from build123d import *

# Parameters (mm, degrees)
SKETCH1_W           = 465.838
SKETCH1_H           = 365.232
BOSS_EXTRUDE1_DEPTH = 3.175
SKETCH2_W           = 465.838
SKETCH2_H           = 365.232
SKETCH2_W_2         = 459.488
SKETCH2_H_2         = 47.625
SKETCH2_W_3         = 89.789
SKETCH2_H_3         = 308.082
SKETCH2_W_4         = 87.632
BOSS_EXTRUDE2_DEPTH = 200.6
SKETCH4_W           = 459.488
SKETCH4_H           = 200.6
CUT_EXTRUDE1_DEPTH  = 3.175
SKETCH5_W           = 89.789
SKETCH5_H           = 308.082
SKETCH5_W_2         = 87.632
BOSS_EXTRUDE5_DEPTH = 38.1
CUT_EXTRUDE2_DEPTH  = 35
BOSS_EXTRUDE6_DEPTH = 50.8
CUT_EXTRUDE3_DEPTH  = 589.161843479
SKETCH10_W          = 34.036
SKETCH10_H          = 101.6
SKETCH10_W_2        = 50.8
SKETCH10_H_2        = 34.036
BOSS_EXTRUDE7_DEPTH = 3.175


with BuildPart() as part:
    # Sketch1 → Boss-Extrude1 (new body)
    with BuildSketch(Plane.XY):
        with Locations((-46.4825, -25.4)):
            Rectangle(SKETCH1_W, SKETCH1_H)
    extrude(amount=BOSS_EXTRUDE1_DEPTH)

    # Sketch2 → Boss-Extrude2 (add)
    with BuildSketch(Plane.XY.offset(3.175)):
        with Locations((-46.4825, -25.4)):
            Rectangle(SKETCH2_W, SKETCH2_H)
        with Locations((-46.4825, -181.0285)):
            Rectangle(SKETCH2_W_2, SKETCH2_H_2, mode=Mode.SUBTRACT)
        with Locations((138.367, 0)):
            Rectangle(SKETCH2_W_3, SKETCH2_H_3, mode=Mode.SUBTRACT)
        with Locations((45.403, 0)):
            Rectangle(SKETCH2_W_3, SKETCH2_H_3, mode=Mode.SUBTRACT)
        with Locations((-47.561, 0)):
            Rectangle(SKETCH2_W_3, SKETCH2_H_3, mode=Mode.SUBTRACT)
        with Locations((-140.525, 0)):
            Rectangle(SKETCH2_W_3, SKETCH2_H_3, mode=Mode.SUBTRACT)
        with Locations((-232.4105, 0)):
            Rectangle(SKETCH2_W_4, SKETCH2_H_3, mode=Mode.SUBTRACT)
    extrude(amount=BOSS_EXTRUDE2_DEPTH)

    # Sketch4 → Cut-Extrude1 (cut)
    with BuildSketch(Plane.XZ.offset(208.016)):
        with Locations((-46.4825, 103.475)):
            Rectangle(SKETCH4_W, SKETCH4_H)
    extrude(amount=-CUT_EXTRUDE1_DEPTH, mode=Mode.SUBTRACT)

    # Sketch5 → Boss-Extrude5 (add)
    with BuildSketch(Plane.XY.offset(203.775)):
        Polygon((186.4365, 157.216), (-279.4015, 157.216), (-279.4015, -208.016), (-276.2265, -208.016), (-276.2265, -157.216), (183.2615, -157.216), (183.2615, -208.016), (186.4365, -208.016), align=None)
        with Locations((-140.525, 0)):
            Rectangle(SKETCH5_W, SKETCH5_H, mode=Mode.SUBTRACT)
        with Locations((-47.561, 0)):
            Rectangle(SKETCH5_W, SKETCH5_H, mode=Mode.SUBTRACT)
        with Locations((45.403, 0)):
            Rectangle(SKETCH5_W, SKETCH5_H, mode=Mode.SUBTRACT)
        with Locations((138.367, 0)):
            Rectangle(SKETCH5_W, SKETCH5_H, mode=Mode.SUBTRACT)
        with Locations((-232.4105, 0)):
            Rectangle(SKETCH5_W_2, SKETCH5_H, mode=Mode.SUBTRACT)
    extrude(amount=BOSS_EXTRUDE5_DEPTH)

    # Sketch7 → Cut-Extrude2 (cut)
    with BuildSketch(Plane.XY.offset(241.875)):
        Polygon((-185.4195, -154.041), (-185.4195, 154.041), (-188.5945, 154.041), (-188.5945, -154.041), (-276.2265, -154.041), (-276.2265, -157.216), (183.2615, -157.216), (183.2615, -154.041), (93.4725, -154.041), (93.4725, 154.041), (90.2975, 154.041), (90.2975, -154.041), (0.5085, -154.041), (0.5085, 154.041), (-2.6665, 154.041), (-2.6665, -154.041), (-92.4555, -154.041), (-92.4555, 154.041), (-95.6305, 154.041), (-95.6305, -154.041), align=None)
    extrude(amount=-CUT_EXTRUDE2_DEPTH, mode=Mode.SUBTRACT)

    # Sketch8 → Boss-Extrude6 (add)
    with BuildSketch(Plane.XY.offset(241.875)):
        Polygon((183.2615, 154.041), (183.2615, -208.016), (186.4365, -208.016), (186.4365, 157.216), (-279.4015, 157.216), (-279.4015, -208.016), (-276.2265, -208.016), (-276.2265, 154.041), align=None)
    extrude(amount=BOSS_EXTRUDE6_DEPTH)

    # Sketch9 → Cut-Extrude3 (cut, through all)
    with BuildSketch(Plane(origin=(186.4365, 0, 0), x_dir=(0, 0, -1), z_dir=(1, 0, 0))):
        Polygon((-292.675, -208.016), (-235.525, -208.016), (-292.675, -131.816), align=None)
        Polygon((-292.675, 157.216), (-292.675, 81.016), (-235.525, 157.216), align=None)
    extrude(amount=-CUT_EXTRUDE3_DEPTH, mode=Mode.SUBTRACT)

    # Sketch10 → Boss-Extrude7 (add)
    with BuildSketch(Plane.XY):
        with Locations((203.4545, 106.416)):
            Rectangle(SKETCH10_W, SKETCH10_H)
        with Locations((203.4545, -106.416)):
            Rectangle(SKETCH10_W, SKETCH10_H)
        with Locations((161.0365, 174.234)):
            Rectangle(SKETCH10_W_2, SKETCH10_H_2)
    boss_extrude7 = extrude(amount=BOSS_EXTRUDE7_DEPTH)

    # Mirror1: Boss-Extrude7 across plane
    add(boss_extrude7.mirror(Plane.ZY.offset(46.4825)))


solid = part.part
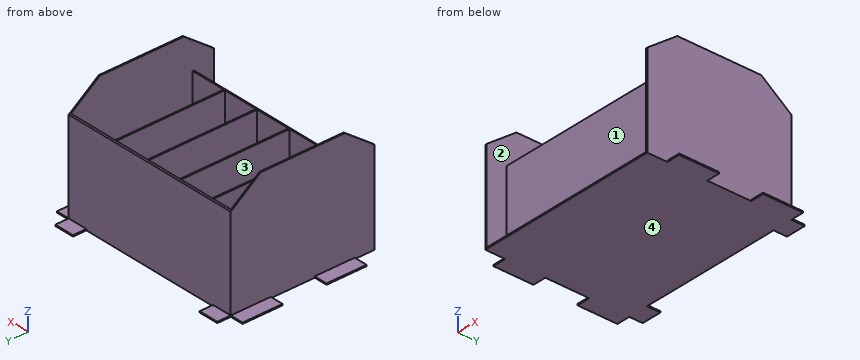
Geometry: final body of the model. Coordinates: model frame, mm. Face numbers are marked on the shaded views. A direction names the side the tool comes from. Give positions to 0.01 mm unless a question says otherwise; leave off trailing zeros. Loops run counter-clockwise (first coordinate to the right, second up) from the corner with the lowest first, then second, coordinate; pieces in that order, holes last. Notation, with made-up numbers: (2, 46.25) - (18, 46.25) arc R26 ccw to (18, 75.25) - close; hole circle Ø1 at (26, 11). An arc over 180 degrees is marked (long way). One line per question, with ' | ' between items. Start each with the question number.
(1) Section query A-A on z = 259. Return loops of the section in (x, y), then the cut area to 3 significant figures.
(2) Contact query for flat-ended pins moving along their axis: pin 1 (5 mm diameter, centred on x = -205, z = 110, fed in from +Y); pin 2 (4 mm diameter, centred on y = 56, z = 255, fed in from -X); pin 3 (10 mm diameter, centred on x = -97.5, y = -90, fed in from +Z) (3 decimals). Output: stop coordinate, or through.
(3) Ray query, line 1 (X direction, y = 75.5, z = 74); line 2 (Y direction, x = -228, z = 92); line 3 (X direction, y = -102, z = 233). Return the intervals inside material, ascending. Write a range as from..to.
(4) Section query C-C on z = 82. Return loops of the section in (x, y).
(5) Reachability of the marked faces 1 and 2 from +Z, -Z, +X, -X, +Y, -Y: full face, straight path, thin tool, end or side. Return the list, or none.
(6) Section query D-D on x = -205.5. Return loops of the section in (y, z) (3 decimals), then the cut area to 3 significant figures.
(7) Section query B-B on y = 37.5. Return loops of the section in (x, z) (1 decimal).
(8) Pull-direction query (X, two-part tool) for the marked faces 3 and 4; classes: released by +X, released by -X, zero draft, split by the parting line, or undercut.
The answers:
1) outline: (-279.4, -176.72) - (-276.23, -176.72) - (-276.23, 125.92) - (-279.4, 125.92) - close; (183.26, -176.72) - (186.44, -176.72) - (186.44, 125.92) - (183.26, 125.92) - close | area: 1,920 mm2
2) pin 1: y = 157.22 | pin 2: x = -279.4 | pin 3: z = 206.875
3) line 1: -279.4..-276.23, -188.59..-185.42, -95.63..-92.46, -2.67..0.51, 90.3..93.47, 183.26..186.44 | line 2: -157.22..-154.04, 154.04..157.22 | line 3: -279.4..-276.23, 183.26..186.44
4) outline: (-279.4, -208.02) - (-276.23, -208.02) - (-276.23, -157.22) - (183.26, -157.22) - (183.26, -208.02) - (186.44, -208.02) - (186.44, 157.22) - (-279.4, 157.22) - close; hole (-276.23, -154.04) - (-188.59, -154.04) - (-188.59, 154.04) - (-276.23, 154.04) - close; hole (-185.42, -154.04) - (-95.63, -154.04) - (-95.63, 154.04) - (-185.42, 154.04) - close; hole (-92.46, -154.04) - (-2.67, -154.04) - (-2.67, 154.04) - (-92.46, 154.04) - close; hole (0.51, -154.04) - (90.3, -154.04) - (90.3, 154.04) - (0.51, 154.04) - close; hole (93.47, -154.04) - (183.26, -154.04) - (183.26, 154.04) - (93.47, 154.04) - close
5) face 1: +Z, -Y | face 2: +Z
6) outline: (-208.016, 0) - (157.216, 0) - (157.216, 235.525) - (154.041, 237.906) - (154.041, 3.175) - (-154.041, 3.175) - (-154.041, 206.875) - (-157.216, 206.875) - (-157.216, 3.175) - (-208.016, 3.175) - close | area: 2,550 mm2
7) outline: (-279.4, 0) - (186.4, 0) - (186.4, 292.7) - (183.3, 292.7) - (183.3, 3.2) - (93.5, 3.2) - (93.5, 206.9) - (90.3, 206.9) - (90.3, 3.2) - (0.5, 3.2) - (0.5, 206.9) - (-2.7, 206.9) - (-2.7, 3.2) - (-92.5, 3.2) - (-92.5, 206.9) - (-95.6, 206.9) - (-95.6, 3.2) - (-185.4, 3.2) - (-185.4, 206.9) - (-188.6, 206.9) - (-188.6, 3.2) - (-276.2, 3.2) - (-276.2, 292.7) - (-279.4, 292.7) - close
8) face 3: undercut | face 4: zero draft
